The listing builds one solid part. Answer for the finished solid, in the listing's coordinates (mm). Face numbers are marked on the shaded views. Round coordinates to 2 decimals unless told otherwise and drop trailing zeros. Order: outer loops, then holes, each group sorted by start corner. A loop starts at its lowest first (then second) coordinate and runs counter-clockwise, first axis right, second up. Notation, with made-up numbers: M 37,-28.75 L 70,-28.75 A36 ccw 70,6.25 Z; hole C 82,47 d3. An arc over 180 degrees is marked long. Write item = value, one per line. Start each with the question number.
(1) A cutting plane is placed at D-D, the plane z = -0.9. Determine the outline of the cut face in (x, y) (3 decimals).
(2) Straight lines are drawn through the part: probe 1 along Y at (x, z) = (0, -4.65) (3 decimals); probe 2 along X at (y, z) = (1.75, -4.5); probe 3 along Z at (x, y) = (3.75, -2.5). For each, find the intervals that lie inside material, in ascending order. Write a range as from..to.
(3) A cutting plane is placed at C-C, the plane x = 3.5. Determine the outline of the cut face in (y, z), and give its area (3 significant figures).
(4) For a pull along Y with two mould halves and no side action, classify the marked faces 1, 2, 3 and 4 as released by +Y, released by -Y, zero draft, split by the parting line, or undercut.
(5) Each of these flat-tipped pins is pushed along its axis until it touches: pin 1 (2 mm diameter, centred on y = -2.5, z = -1, fed in from +X); pin 2 (1.5 mm diameter, centred on y = 4.5, z = -0.5, fed in from +X); pin 3 (1.5 mm diameter, centred on y = 3, z = -3.5, fed in from -X). Where does it stop, or does it pass through?
Autodesk Inventor part; units mm, degrees
ref_plane "YZ Plane" through (0, 0, 0) normal (1, 0, 0) x (0, 1, 0)
ref_plane "XZ Plane" through (0, 0, 0) normal (0, 1, 0) x (-1, 0, 0)
ref_plane "XY Plane" through (0, 0, 0) normal (0, 0, 1) x (1, 0, 0)
sketch "Sketch1" plane through (0, 0, 0) normal (0, 0, 1) x (1, 0, 0)
  circle A0 centre (0, 0) radius 3.175
  circle A1 centre (0, 0) radius 6.35
  dimension "d0" = 6.35
  dimension "d1" = 12.7
extrude "Extrusion1" add sketch "Sketch1" against normal blind 4.7625
sketch "Sketch2" plane through (0, 0, 0) normal (0, 0, 1) x (1, 0, 0)
  circle A0 centre (0, 0) radius 6.35
  circle A1 centre (0, 0) radius 3.175
  circle A2 centre (0, 0) radius 5.715
  circle A3 centre (0, 0) radius 3.81
  dimension "d4" = 0.635
  dimension "d5" = 0.635
extrude "Extrusion2" cut sketch "Sketch2" against normal blind 0.381 contours A2
sketch "Sketch3" plane through (0, 0, -4.7625) normal (0, 0, -1) x (-1, 0, 0)
  circle A0 centre (0, 0) radius 5.715
  circle A1 centre (0, 0) radius 3.81
extrude "Extrusion3" cut sketch "Sketch3" against normal blind 0.381
properties part number "0.25in ID 0.5in OD 0.1875in Deep Roller Bearing"
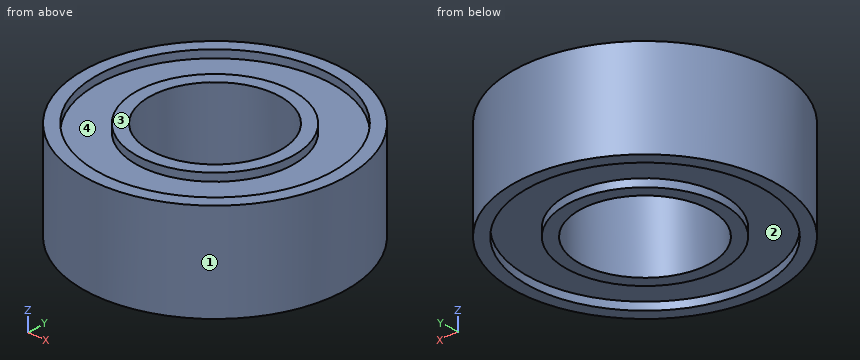
Reported:
q1.outline = C 0,0 d12.7; hole C 0,0 d6.35
q2.probe_1 = -6.35..-5.715, -3.81..-3.175, 3.175..3.81, 5.715..6.35
q2.probe_2 = -6.1..-5.44, -3.38..-2.65, 2.65..3.38, 5.44..6.1
q2.probe_3 = -4.38..-0.38
q3.outline = M -5.3,-4.76 L -4.52,-4.76 L -4.52,-4.38 L -1.51,-4.38 L -1.51,-4.76 L 1.51,-4.76 L 1.51,-4.38 L 4.52,-4.38 L 4.52,-4.76 L 5.3,-4.76 L 5.3,0 L 4.52,0 L 4.52,-0.38 L 1.51,-0.38 L 1.51,0 L -1.51,0 L -1.51,-0.38 L -4.52,-0.38 L -4.52,0 L -5.3,0 Z
q3.area = 45.9 mm²
q4.face_1 = split by the parting line
q4.face_2 = undercut
q4.face_3 = zero draft
q4.face_4 = undercut
q5.pin_1 = 6.17
q5.pin_2 = 5.12
q5.pin_3 = -5.94
